Could you check a few things on this model? Use its own coordinates, in mm. Give positions to 0.01 mm unless a question says otherwise; leave off trailing zeros. Write each loop counter-clockwise with the first axis right and the second up, starting at its lowest first coordinate (ties: lowest second). Pieces come first, ordered by that corner, then holes. Notation, with made-up numbers: (12.5, 61.25) - (36.5, 61.25) arc R19 ccw to (36.5, 70.25) - close; hole circle Ø3 at (-2.5, 4.25). An arc over 180 degrees is marked (long way). Use one line per item in the form item = value.
```python
from build123d import *

# Parameters (mm, degrees)
SWEEP1_PROFILE_R = 15
SHELL1_T         = -2


with BuildPart() as part:
    # Sweep1: sweep along a path in Sketch1
    with BuildLine(Plane(origin=(0, 0, 0), x_dir=(1, 0, 0), z_dir=(0, 1, 0))) as sweep1_path:
        Line((-50, 0), (-17, 0))
        ThreePointArc((-17, 0), (-4.97918472, 4.97918472), (0, 17))
        Line((0, 17), (0, 50))
    # Sweep1 profile (on start of the path) → Sweep1 (sweep)
    with BuildSketch(Plane(origin=(-50, 0, 0), x_dir=(0, 0, 1), z_dir=(1, 0, 0))):
        Circle(SWEEP1_PROFILE_R)
    sweep(path=sweep1_path.line)

    # Shell1
    shell1_openings = [part.faces().sort_by_distance(p)[0] for p in [
        (0, 0, -50),
        (-50, 0, 0),
    ]]
    offset(amount=SHELL1_T, openings=shell1_openings, kind=Kind.INTERSECTION)


solid = part.part
```
1. Imagine slicing it at A-A, the plane y = 0. List the corners of the cut face in (x, z) for me.
Response values:
outline = (-50, -15) - (-17, -15) arc R2 cw to (-15, -17) - (-15, -50) - (-13, -50) - (-13, -17) arc R4 ccw to (-17, -13) - (-50, -13) - close; (-50, 13) - (-17, 13) arc R30 cw to (13, -17) - (13, -50) - (15, -50) - (15, -17) arc R32 ccw to (-17, 15) - (-50, 15) - close
2. If we mould it in two halves opening along Z, with no side actions, what happens to faces 1 (the face through (-50, -13.4, -0.1)), 2 (the face through (-33.269, -0.66, -14.985)), 3 (the face through (-33.269, 7.91, -10.316)), 4 (the face through (0.1, 13.4, -50))? For each: pulls with the +Z half, pulls with the -Z half, needs draft (parallel to the pull), parting line crosses it, or undercut.
Response values:
face_1 = needs draft
face_2 = parting line crosses it
face_3 = undercut
face_4 = pulls with the -Z half
3. If I drill on line 1 (Y direction, x = 0, z = -42), over which ranges is the centre line in solid material (lowest first)? Write a range as from..to.
Response values:
line_1 = -15..-13, 13..15
4. Imagine slicing it at C-C, the plane y = 7.5. List the corners of the cut face in (x, z) for me, and give its area (3 significant figures).
Response values:
outline = (-50, -12.99) - (-17, -12.99) arc R4.01 cw to (-12.99, -17) - (-12.99, -50) - (-10.62, -50) - (-10.62, -17) arc R6.38 ccw to (-17, -10.62) - (-50, -10.62) - close; (-50, 10.62) - (-17, 10.62) arc R27.62 cw to (10.62, -17) - (10.62, -50) - (12.99, -50) - (12.99, -17) arc R29.99 ccw to (-17, 12.99) - (-50, 12.99) - close
area = 440 mm²
5. For pin 1 (1 mm diameter, centred on x = -33.5, y = 3, fed in from -Z); pin 2 (12 mm diameter, centred on x = 7, z = -20, fed in from -Y); pin 3 (1 mm diameter, centred on y = 8, z = -20, fed in from +X), each with a flat end and sliding along its axis, tell me the tip position at first contact or that it passes through.
Response values:
pin_1 = -14.79
pin_2 = -14.97
pin_3 = 12.99
6. Imagine slicing it at B-B, the plane z = -32. List the corners of the cut face in (x, y) for me, and give its area (3 significant figures).
Response values:
outline = circle Ø30 at (0, 0); hole circle Ø26 at (0, 0)
area = 176 mm²
